Build history of the part. All positions in model axes, mm. A direction names the side the tool comes from. Give positions to 0.01 mm unless a question says otherwise; leave off trailing zeros. Loops run counter-clockwise (first coordinate to the right, second up) from the corner with the lowest first, then second, coordinate; pieces in that order, holes last. Notation, with made-up numbers: (68.25, -17) - (80.25, -17) arc R27 cw to (80.25, 2) - close; hole circle Ø2 at (-1.5, 38). An arc over 180 degrees is marked (long way). Return JSON: item names as keys, results as strings. Group by question number.
1) Slice it at A-A (z = 4.75). List the corners of the cut face in (x, y) (3 decimals).
2) Drill centre lines: probe 1 along Y at (x, z) = (0, 4.25) (3 decimals); probe 2 along Y at (x, z) = (0, 7.75) (3 decimals); probe 3 along Z at (x, y) = (-9, -2). Where is each one in solid material? Low to high. Write a range as from..to.
3) Slice it at C-C (y = 0.5). Count the separate pieces of the cut face and the enclosed holes in it, and give its area (3 significant figures).
4) Drop a flat-ended pin along its axis: pin 1 (3 mm diameter, centred on x = 6.5, y = -5.5, fed in from +Z). Give the stop position or say it passes through.
5) Slice it at B-B (x = 0). List the corners of the cut face in (y, z) (3 decimals).
6) 3-axis set-ups, long thin cutter, end or side, ignore diameter. For faces 4 (the face through (0.5, 0, 1)), 5 (the face through (-3.746, 0.165, 8.606)), 6 (the face through (1, 2, 10)): which of +Z, -Z, +X, -X, +Y, -Y reach the whole face in a straight line?
7) Mould opens along X. For faces 1 (the face through (-0.5, 0, 1)), 2 (the face through (0, 0, 0)), 3 (the face through (-2.17, -9.76, 3.08)) say: released by +X, released by -X, zero draft, split by the parting line, or undercut.
8) Slice it at D-D (y = -8.25). List the corners of the cut face in (x, z), and give its area (3 significant figures).
```python
from build123d import *

# Parameters (mm, degrees)
SKETCH1_R           = 10
BOSS_EXTRUDE1_DEPTH = 1.25
SKETCH2_R           = 10
SKETCH2_R_2         = 1.875
BOSS_EXTRUDE2_DEPTH = 5
SKETCH3_R           = 3.75
SKETCH3_R_2         = 1.875
BOSS_EXTRUDE3_DEPTH = 3.75
FILLET1_R           = 1


with BuildPart() as part:
    # Sketch1 → Boss-Extrude1 (new body)
    with BuildSketch(Plane.XY):
        Circle(SKETCH1_R)
        with BuildLine():
            Line((-0.5, 1.807104037), (-0.5, -1.807104037))
            ThreePointArc((-0.5, -1.807104037), (-1.875, 0), (-0.5, 1.807104037))
        make_face(mode=Mode.SUBTRACT)
        with BuildLine():
            Line((0.5, 1.807104037), (0.5, -1.807104037))
            ThreePointArc((0.5, -1.807104037), (1.875, 0), (0.5, 1.807104037))
        make_face(mode=Mode.SUBTRACT)
    extrude(amount=BOSS_EXTRUDE1_DEPTH)

    # Sketch2 → Boss-Extrude2 (add)
    with BuildSketch(Plane.XY.offset(1.25)):
        Circle(SKETCH2_R)
        Circle(SKETCH2_R_2, mode=Mode.SUBTRACT)
    extrude(amount=BOSS_EXTRUDE2_DEPTH)

    # Sketch3 → Boss-Extrude3 (add)
    with BuildSketch(Plane.XY.offset(6.25)):
        Circle(SKETCH3_R)
        Circle(SKETCH3_R_2, mode=Mode.SUBTRACT)
    extrude(amount=BOSS_EXTRUDE3_DEPTH)

    # Fillet1
    fillet1_edges = [part.edges().sort_by_distance(p)[0] for p in [
        (-3.75, 0, 6.25),
    ]]
    fillet(fillet1_edges, radius=FILLET1_R)


solid = part.part
```
Results:
{
 "1": {"outline": "circle Ø20 at (0, 0); hole circle Ø3.75 at (0, 0)"},
 "2": {"probe 1": "-10..-1.875, 1.875..10", "probe 2": "-3.75..-1.875, 1.875..3.75", "probe 3": "0..6.25"},
 "3": {"separate pieces": "3", "enclosed holes": "0", "area": "118 mm2"},
 "4": {"pin 1": "z = 6.25"},
 "5": {"outline": "(-10, 0) - (10, 0) - (10, 6.25) - (4.75, 6.25) arc R1 cw to (3.75, 7.25) - (3.75, 10) - (1.875, 10) - (1.875, 1.25) - (-1.875, 1.25) - (-1.875, 10) - (-3.75, 10) - (-3.75, 7.25) arc R1 cw to (-4.75, 6.25) - (-10, 6.25) - close"},
 "6": {"face 4": "+Z, -Z", "face 5": "+Z", "face 6": "+Z, +X, -X, +Y, -Y"},
 "7": {"face 1": "undercut", "face 2": "zero draft", "face 3": "split by the parting line"},
 "8": {"outline": "(-5.65, 0) - (5.65, 0) - (5.65, 6.25) - (-5.65, 6.25) - close", "area": "70.6 mm2"}
}
